```python
from build123d import *

# Parameters (mm, degrees)
F0_W     = 25
F0_H     = 12.5
F0_R     = 3.25
F0_R_2   = 2.5
F1_DEPTH = 25
F2_T     = -1
F3_DEPTH = 10
F4_DEPTH = 5
F5_R     = 3.3
F6_DEPTH = 10
F5_R_2   = 4.5
F7_DEPTH = 5
F8_R     = 1


# Not quite as in the source:
# - a fillet or chamfer that OpenCascade refuses, or shapes differently, is made with other operations: its cross-section is extruded or revolved along the edge and cut away or added


with BuildPart() as f1:
    # F0 (on Front) → F1 (new body)
    with BuildSketch(Plane.XZ):
        with Locations((1.7170939115, 9.0107331052)):
            Rectangle(F0_W, F0_H)
        with Locations((-3.0594504727, 9.0107331052)):
            Circle(F0_R, mode=Mode.SUBTRACT)
        with Locations((6.4404988661, 9.0417582542)):
            Circle(F0_R, mode=Mode.SUBTRACT)
        with Locations((-3.0594504727, 9.0107331052)):
            Circle(F0_R)
        with Locations((-3.0594504727, 9.0107331052)):
            Circle(F0_R_2, mode=Mode.SUBTRACT)
        with Locations((6.4404988661, 9.0417582542)):
            Circle(F0_R)
        with Locations((6.4404988661, 9.0417582542)):
            Circle(F0_R_2, mode=Mode.SUBTRACT)
        with Locations((-3.0594504727, 9.0107331052)):
            Circle(F0_R_2)
        with Locations((6.4404988661, 9.0417582542)):
            Circle(F0_R_2)
    extrude(amount=F1_DEPTH)

    # F2
    f2_openings = [f1.faces().sort_by_distance(p)[0] for p in [
        (1.717094, -12.5, 2.760733),
    ]]
    offset(amount=F2_T, openings=f2_openings)

    # F0 (on Front) → F3 (cut)
    with BuildSketch(Plane.XZ):
        with Locations((6.4404988661, 9.0417582542)):
            Circle(F0_R_2)
        with Locations((-3.0594504727, 9.0107331052)):
            Circle(F0_R_2)
    extrude(amount=F3_DEPTH, mode=Mode.SUBTRACT)

    # F0 (on Front) → F4 (join)
    with BuildSketch(Plane.XZ):
        with Locations((-3.0594504727, 9.0107331052)):
            Circle(F0_R)
        with Locations((-3.0594504727, 9.0107331052)):
            Circle(F0_R_2, mode=Mode.SUBTRACT)
        with Locations((6.4404988661, 9.0417582542)):
            Circle(F0_R)
        with Locations((6.4404988661, 9.0417582542)):
            Circle(F0_R_2, mode=Mode.SUBTRACT)
    extrude(amount=-F4_DEPTH)

    # F5 (on face) → F6 (cut)
    with BuildSketch(Plane.XZ.offset(25)):
        with Locations((-3.2763871515, 8.743028397)):
            Circle(F5_R)
        with Locations((8.7236128485, 8.743028397)):
            Circle(F5_R)
    extrude(amount=-F6_DEPTH, mode=Mode.SUBTRACT)

    # F5 (on face) → F7 (join)
    with BuildSketch(Plane.XZ.offset(25)):
        with Locations((-3.2763871515, 8.743028397)):
            Circle(F5_R_2)
        with Locations((-3.2763871515, 8.743028397)):
            Circle(F5_R, mode=Mode.SUBTRACT)
        with Locations((8.7236128485, 8.743028397)):
            Circle(F5_R_2)
        with Locations((8.7236128485, 8.743028397)):
            Circle(F5_R, mode=Mode.SUBTRACT)
    extrude(amount=F7_DEPTH)

    # F8
    f8_edges = [f1.edges().sort_by_distance(p)[0] for p in [
        (14.217094, -25, 9.010733),
        (14.217094, -12.5, 15.260733),
        (1.717094, -25, 15.260733),
        (-10.782906, -25, 9.010733),
        (14.217094, 0, 9.010733),
        (1.717094, 0, 15.260733),
        (-10.782906, 0, 9.010733),
        (-10.782906, -12.5, 15.260733),
    ]]
    fillet(f8_edges, radius=F8_R)

    # F9: fillet of radius 1 on 4 edges, made by hand

    # F9_s1 → F9_t2 (revolve, cut)
    with BuildSketch(Plane.XY.offset(9.0417582542)):
        with BuildLine():
            ThreePointArc((9.6906488661, 4.0318703599), (9.4811826994, 4.6442887287), (8.9405363493, 5.0001452412))
            Line((8.9405363493, 5.0001452412), (8.9455340989, 5.0195107389))
            ThreePointArc((8.9455340989, 5.0195107389), (9.3155176077, 5.02), (9.6904988661, 5.02))
            Line((9.6904988661, 5.02), (9.7104988661, 5))
            ThreePointArc((9.7104988661, 5), (9.7104988661, 4.51593518), (9.7106488661, 4.0318703599))
            Line((9.7106488661, 4.0318703599), (9.6906488661, 4.0318703599))
        make_face()
    revolve(axis=Axis((6.4404988661, 5, 9.0417582542), (0, -1, 0)), mode=Mode.SUBTRACT)

    # F9_s3 → F9_t4 (revolve, cut)
    with BuildSketch(Plane.XY.offset(9.0107331052)):
        with BuildLine():
            ThreePointArc((0.1906995273, 4.0318703599), (-0.0187666394, 4.6442887287), (-0.5594129896, 5.0001452412))
            Line((-0.5594129896, 5.0001452412), (-0.5544152399, 5.0195107389))
            ThreePointArc((-0.5544152399, 5.0195107389), (-0.1844317311, 5.02), (0.1905495273, 5.02))
            Line((0.1905495273, 5.02), (0.2105495273, 5))
            ThreePointArc((0.2105495273, 5), (0.2105495273, 4.51593518), (0.2106995273, 4.0318703599))
            Line((0.2106995273, 4.0318703599), (0.1906995273, 4.0318703599))
        make_face()
    revolve(axis=Axis((-3.0594504727, 5, 9.0107331052), (0, -1, 0)), mode=Mode.SUBTRACT)

    # F9_s5 → F9_t6 (revolve, cut)
    with BuildSketch(Plane.XY.offset(8.743028397)):
        with BuildLine():
            ThreePointArc((1.2237628485, -29.00015), (0.9308696297, -29.7072567812), (0.2237628485, -30.00015))
            Line((0.2237628485, -30.00015), (0.2237628485, -30.02015))
            ThreePointArc((0.2237628485, -30.02015), (0.7236878485, -30.02), (1.2236128485, -30.02))
            Line((1.2236128485, -30.02), (1.2436128485, -30))
            ThreePointArc((1.2436128485, -30), (1.2436128485, -29.500075), (1.2437628485, -29.00015))
            Line((1.2437628485, -29.00015), (1.2237628485, -29.00015))
        make_face()
    revolve(axis=Axis((-3.2763871515, -30, 8.743028397), (0, -1, 0)), mode=Mode.SUBTRACT)

    # F9_s7 → F9_t8 (revolve, cut)
    with BuildSketch(Plane.XY.offset(8.743028397)):
        with BuildLine():
            ThreePointArc((13.2237628485, -29.00015), (12.9308696297, -29.7072567812), (12.2237628485, -30.00015))
            Line((12.2237628485, -30.00015), (12.2237628485, -30.02015))
            ThreePointArc((12.2237628485, -30.02015), (12.7236878485, -30.02), (13.2236128485, -30.02))
            Line((13.2236128485, -30.02), (13.2436128485, -30))
            ThreePointArc((13.2436128485, -30), (13.2436128485, -29.500075), (13.2437628485, -29.00015))
            Line((13.2437628485, -29.00015), (13.2237628485, -29.00015))
        make_face()
    revolve(axis=Axis((8.7236128485, -30, 8.743028397), (0, -1, 0)), mode=Mode.SUBTRACT)


solid = f1.part
```
Input: part model. Units: mm. Frame: model coordinates. A direction names the side the tool comes from. Round coordinates to 2 decimals unless told otherwise and drop trailing zeros. Loops run counter-clockwise (first coordinate to the right, second up) from the corner with the lowest first, then second, coordinate; pieces in that order, holes last. Notation, with made-up numbers: M -5.75,9 L 21.25,9 A27 ccw 21.25,39 Z; hole C -9.75,-38.5 d7. An arc over 180 degrees is marked long. Answer in a Markdown table with one row per item. Add a question column.
1. Set-up query: faces 4 (the face through (4.598, 2.042, 10.731)), 5 (the face through (-10.482, -24.715, 8.591)), 6 (the face through (-9.783, -12, 8)), 7 (the face through (4.228, -26.981, 8.941)). Return all of +Z, -Z, +X, -X, +Y, -Y with unobstructed straight access to the full face (end or side cutting, diameter ignored); none if empty.
2. Section D-D (x = -2.75). Give the number of separate pieces and of enclosed holes in the cut face, and give its area (3 significant figures).
3. Section C-C (y = -27). Output: boundary loops of the cut face in (x, z).
4. Section B-B (y = -15). Output: boundary loops of the cut face in (x, z).
5. Ray query, probe 1 along Y at (x, z) = (3, 8.5); probe 2 along Z at (x, y) = (-9.5, -16); probe 3 along X at (y, z) = (-22.5, 6.5). Return the intervals inside material, ascending.
6. Contact query for flat-ended pins moving along their axis: pin 1 (7 mm diameter, centred on x = -3.5, y = -15.5, fed in from -Z); pin 2 (6.5 mm diameter, centred on x = -3.06, z = 9.01, fed in from +Y); pin 3 (3 mm diameter, centred on x = 6.44, z = 9.04, fed in from +Y); pin 4 (6 mm diameter, centred on x = 8.72, z = 8.74, fed in from -Y). Output: stop coordinate, or through.
7. Section A-A (x = -9). Output: boundary loops of the cut face in (y, z), and give its area (3 significant figures).
8. Mould query, pull axis X, two halves, no side actions, for faces 1 (the face through (2, -12, 15.261)), 2 (the face through (-10.783, -12, 8)), 3 (the face through (2, -25, 9)). Classes: released by +X, released by -X, zero draft, split by the parting line, or undercut.
Values follow:
| question | item | result |
|---|---|---|
| 1 | face 4 | +Y |
| 1 | face 5 | +Z, -Z, -X, -Y |
| 1 | face 6 | -Z |
| 1 | face 7 | -Y |
| 2 | separate pieces | 3 |
| 2 | enclosed holes | 0 |
| 2 | area | 54.9 mm^2 |
| 3 | outline | C -3.28,8.74 d9; C 8.72,8.74 d9; hole C -3.28,8.74 d6.6; hole C 8.72,8.74 d6.6 |
| 4 | outline | M -10.78,2.76 L -9.78,2.76 L -9.78,14.26 L 13.22,14.26 L 13.22,2.76 L 14.22,2.76 L 14.22,14.26 A1 ccw 13.22,15.26 L -9.78,15.26 A1 ccw -10.78,14.26 Z |
| 5 | probe 1 | -25 to -24, -1 to 0 |
| 5 | probe 2 | 14.26 to 15.26 |
| 5 | probe 3 | -10.78 to -9.78, 13.22 to 14.22 |
| 6 | pin 1 | z = 14.26 |
| 6 | pin 2 | y = 5 |
| 6 | pin 3 | y = -24 |
| 6 | pin 4 | y = -1 |
| 7 | outline | M -25,2.76 L -24,2.76 L -24,14.26 L -1,14.26 L -1,2.76 L 0,2.76 L 0,14.26 A1 ccw -1,15.26 L -24,15.26 A1 ccw -25,14.26 Z |
| 7 | area | 47.6 mm^2 |
| 8 | face 1 | zero draft |
| 8 | face 2 | released by -X |
| 8 | face 3 | undercut |
